from build123d import *

# Parameters (mm, degrees)
SKETCH_W     = 53.34
SKETCH_H     = 20.32
PAD_DEPTH    = 1.6
SKETCH001_R  = 0.45
POCKET_DEPTH = 5


with BuildPart() as part:
    # Sketch → Pad (new body)
    with BuildSketch(Plane.XY):
        Rectangle(SKETCH_W, SKETCH_H)
    extrude(amount=-PAD_DEPTH)

    # Sketch001 (on Face5 of Pad) → Pocket (cut)
    with BuildSketch(Plane.XY):
        with Locations((-24.13, 7.62)):
            Circle(SKETCH001_R)
        with Locations((-21.59, 7.619987)):
            Circle(SKETCH001_R)
        with Locations((-19.05, 7.619987)):
            Circle(SKETCH001_R)
        with Locations((-16.51, 7.619987)):
            Circle(SKETCH001_R)
        with Locations((-13.97, 7.619987)):
            Circle(SKETCH001_R)
        with Locations((-11.43, 7.619987)):
            Circle(SKETCH001_R)
        with Locations((-8.89, 7.619987)):
            Circle(SKETCH001_R)
        with Locations((-6.35, 7.619987)):
            Circle(SKETCH001_R)
        with Locations((-3.81, 7.619987)):
            Circle(SKETCH001_R)
        with Locations((-1.27, 7.619987)):
            Circle(SKETCH001_R)
        with Locations((1.27, 7.619987)):
            Circle(SKETCH001_R)
        with Locations((3.81, 7.619987)):
            Circle(SKETCH001_R)
        with Locations((6.35, 7.619987)):
            Circle(SKETCH001_R)
        with Locations((8.89, 7.619987)):
            Circle(SKETCH001_R)
        with Locations((11.43, 7.619987)):
            Circle(SKETCH001_R)
        with Locations((13.97, 7.619987)):
            Circle(SKETCH001_R)
        with Locations((16.51, 7.619987)):
            Circle(SKETCH001_R)
        with Locations((19.05, 7.619987)):
            Circle(SKETCH001_R)
        with Locations((21.59, 7.619987)):
            Circle(SKETCH001_R)
        with Locations((24.13, 7.619987)):
            Circle(SKETCH001_R)
        with Locations((-24.13, -7.62)):
            Circle(SKETCH001_R)
        with Locations((-21.59, -7.62)):
            Circle(SKETCH001_R)
        with Locations((-19.05, -7.62)):
            Circle(SKETCH001_R)
        with Locations((-16.51, -7.62)):
            Circle(SKETCH001_R)
        with Locations((-13.97, -7.62)):
            Circle(SKETCH001_R)
        with Locations((-11.43, -7.62)):
            Circle(SKETCH001_R)
        with Locations((-8.89, -7.62)):
            Circle(SKETCH001_R)
        with Locations((-6.35, -7.62)):
            Circle(SKETCH001_R)
        with Locations((-3.81, -7.62)):
            Circle(SKETCH001_R)
        with Locations((-1.27, -7.62)):
            Circle(SKETCH001_R)
        with Locations((1.27, -7.62)):
            Circle(SKETCH001_R)
        with Locations((3.81, -7.62)):
            Circle(SKETCH001_R)
        with Locations((6.35, -7.62)):
            Circle(SKETCH001_R)
        with Locations((8.89, -7.62)):
            Circle(SKETCH001_R)
        with Locations((11.43, -7.62)):
            Circle(SKETCH001_R)
        with Locations((13.97, -7.62)):
            Circle(SKETCH001_R)
        with Locations((16.51, -7.62)):
            Circle(SKETCH001_R)
        with Locations((19.05, -7.62)):
            Circle(SKETCH001_R)
        with Locations((21.59, -7.62)):
            Circle(SKETCH001_R)
        with Locations((24.13, -7.62)):
            Circle(SKETCH001_R)
        with Locations((20.32, 3.81)):
            Circle(SKETCH001_R)
        with Locations((20.32, 1.27)):
            Circle(SKETCH001_R)
        with Locations((20.32, -1.27)):
            Circle(SKETCH001_R)
        with Locations((20.32, -3.81)):
            Circle(SKETCH001_R)
    extrude(amount=-POCKET_DEPTH, mode=Mode.SUBTRACT)


solid = part.part
Read the model definition and answer for the solid it produces. Units are mm, in the model's axes. Round coordinates to 2 decimals unless told otherwise and drop trailing zeros. One line per question, with ' | ' between items. Start each with the question number.
Q1. Section A-A on z = -0.7 is taken. Count the separate pieces of the cut face and the enclosed holes in it, plus the area to 3 significant figures.
Q2. For a pull along X with two mould halves and no side action, classify faces 1 (the flat face through (26.67, 0, -1)), 2 (the cylindrical face through (10.98, 7.64, -0.79)) as +X half, -X half, draft (parallel to the pull), parting line (faces both ways), or undercut.
Q3. Find the intervals of material crossed by L1, parallel to Y at x = -14, z = -0.2; L2, parallel to X at y = -1.25, z = -0.75; L3, parallel to Y at x = 20, z = -1.4, in increasing order.
Established:
1) separate pieces: 1 | enclosed holes: 44 | area: 1,060 mm²
2) face 1: +X half | face 2: undercut
3) L1: -10.16 to -8.07, -7.17 to 7.17, 8.07 to 10.16 | L2: -26.67 to 19.87, 20.77 to 26.67 | L3: -10.16 to -4.13, -3.49 to -1.59, -0.95 to 0.95, 1.59 to 3.49, 4.13 to 10.16
